Verification items for the finished model (mm, model axes). A direction names the side the tool comes from. Coordinates: 2 decimals unless noted, no trailing zeros.
Q1. Draft check along Z on faces 4 (the flat face through (-9.525, -62.1, 6.5)), 5 (the flat face through (-3.175, -47, 0)), 6 (the flat face through (0, -48, -9.525)). Enter one of: pulls with the +Z half, pulls with the -Z half, needs draft (parallel to the pull), parting line crosses it, or undercut.
Q2. Thickness scan on line 1 (Z direction, x = 5.5, y = -32) (3 decimals); line 2 (X direction, y = -33, z = 5) (3 decimals); line 3 (Z direction, x = 2.5, y = -45) (3 decimals). Record the ranges inside material, lowest first.
Q3. Set-up check for faces 1 (the flat face through (3.175, -47, 0)), 2 (the flat face through (-6, -69.85, 0)), 3 (the flat face through (0, -69.85, 22)): record each of +Z, -Z, +X, -X, +Y, -Y from which the full face is reachable in a straight line by a thin tool's end or side.
Q4. Depth check by flat-ended pin: P1, Ø3, axis at x = -7.5, z = 2.5, coming from the +Y side; P2, Ø1.9, axis at x = 7, y = -48, coming from the +Z side (3 decimals); P3, Ø8, axis at x = -10.5, y = 9, coming from the -Z side. Enter the tip coordinate at first touch or a pass-through.
from build123d import *

# Parameters (mm, degrees)
F2_W     = 19.05
F2_H     = 19.05
F3_DEPTH = 76.2
F4_W     = 19.05
F4_H     = 6.35
F5_DEPTH = 25.4
F7_DEPTH = 6.35
F10_F1_R = 1.5875
F10_F2_R = 1.5875


with BuildPart() as f1:
    # F0 (on Top) → F1 (revolve)
    with BuildSketch(Plane.XY):
        with BuildLine():
            Line((0, -25.4), (0, 25.4))
            ThreePointArc((0, 25.4), (-25.4, 0), (0, -25.4))
        make_face()
    revolve(axis=Axis((0, -0.8307937533, 0), (0, 1, 0)))

    # F2 (on Front) → F3 (join)
    with BuildSketch(Plane.XZ):
        Rectangle(F2_W, F2_H)
    extrude(amount=F3_DEPTH)

    # F4 (on face) → F5 (join)
    with BuildSketch(Plane.XY.offset(9.525)):
        with Locations((0, -73.025)):
            Rectangle(F4_W, F4_H)
    extrude(amount=F5_DEPTH)


with BuildPart() as f7:
    # F6 (on face) → F7 (new body, symmetric)
    with BuildSketch(Plane.YZ.offset(9.525)):
        with BuildLine():
            Line((-22.6740352606, 6.35), (-69.85, 6.35))
            Line((-69.85, 6.35), (-69.85, -6.35))
            Line((-69.85, -6.35), (-22.6740352606, -6.35))
            ThreePointArc((-22.6740352606, -6.35), (-23.5464301965, 0), (-22.6740352606, 6.35))
        make_face()
    extrude(amount=F7_DEPTH, both=True)


with BuildPart() as f8_1:
    # F8: instance of F7
    add(f7.part.mirror(Plane.YZ))


with BuildPart() as f1_1:
    add(f1.part)

    # F9: cut F8_1, F7
    add(f8_1.part, mode=Mode.SUBTRACT)
    add(f7.part, mode=Mode.SUBTRACT)

    # F10: fillet of radius 1.5875 on 12 edges, made by hand

    # F10_f1
    f10_f1_edges = [f1_1.edges().sort_by_distance(p)[0] for p in [
        (0, -69.85, 9.525),
    ]]
    fillet(f10_f1_edges, radius=F10_F1_R)

    # F10_f2
    f10_f2_edges = [f1_1.edges().sort_by_distance(p)[0] for p in [
        (0, -76.2, 34.925),
        (9.525, -73.025, 34.925),
        (0, -69.85, 34.925),
        (-9.525, -73.025, 34.925),
        (9.525, -76.2, 12.7),
        (-9.525, -76.2, 12.7),
        (-9.525, -69.85, 23.01875),
        (9.525, -69.85, 23.01875),
        (0, -76.2, -9.525),
        (9.525, -48.8669488482, -9.525),
        (-9.525, -48.8669488482, -9.525),
        (9.525, -69.3850320151, 9.9899679849),
        (-9.525, -69.3850320151, 9.9899679849),
    ]]
    fillet(f10_f2_edges, radius=F10_F2_R)


solid = f1_1.part
Check values:
1. face 4: needs draft
1. face 5: undercut
1. face 6: pulls with the -Z half
2. line 1: z = -9.525 to -6.35, 6.35 to 9.525
2. line 2: x = -3.175 to 3.175
2. line 3: z = -9.525 to 9.525
3. face 1: +X
3. face 2: -X
3. face 3: +Z, +X, -X
4. P1: stops at y = 24.58
4. P2: stops at z = 9.525
4. P3: stops at z = -23.42
